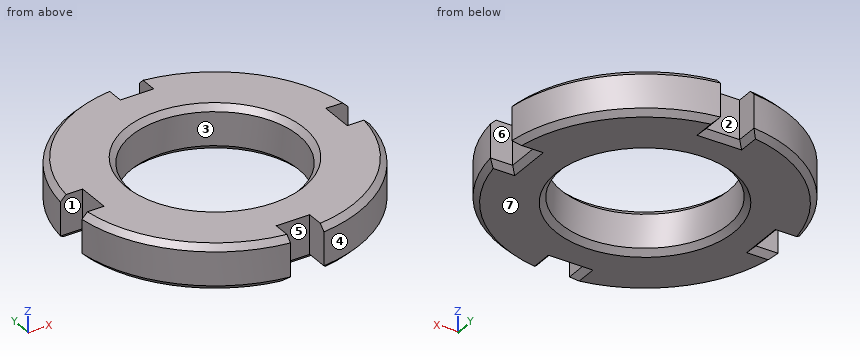
```python
from build123d import *

# Parameters (mm, degrees)
SKETCH_1_R      = 7.5
EXTRUDE_1_DEPTH = 4
CHAMFER_1_SIZE  = 0.5


with BuildPart() as part:
    # Эскиз1 → Бобышка-Вытянуть1 (new body)
    with BuildSketch(Plane.XY):
        with BuildLine():
            Line((1.5, 12.91317157), (1.5, 10.91317157))
            Line((1.5, 10.91317157), (-1.5, 10.91317157))
            Line((-1.5, 10.91317157), (-1.5, 12.91317157))
            ThreePointArc((-1.5, 12.91317157), (-9.192388155, 9.192388155), (-12.91317157, 1.5))
            Line((-12.91317157, 1.5), (-10.91317157, 1.5))
            Line((-10.91317157, 1.5), (-10.91317157, -1.5))
            Line((-10.91317157, -1.5), (-12.91317157, -1.5))
            ThreePointArc((-12.91317157, -1.5), (-9.192388155, -9.192388155), (-1.5, -12.91317157))
            Line((-1.5, -12.91317157), (-1.5, -10.91317157))
            Line((-1.5, -10.91317157), (1.5, -10.91317157))
            Line((1.5, -10.91317157), (1.5, -12.91317157))
            ThreePointArc((1.5, -12.91317157), (9.192388155, -9.192388155), (12.91317157, -1.5))
            Line((12.91317157, -1.5), (10.91317157, -1.5))
            Line((10.91317157, -1.5), (10.91317157, 1.5))
            Line((10.91317157, 1.5), (12.91317157, 1.5))
            ThreePointArc((12.91317157, 1.5), (9.192388155, 9.192388155), (1.5, 12.91317157))
        make_face()
        Circle(SKETCH_1_R, mode=Mode.SUBTRACT)
    extrude(amount=EXTRUDE_1_DEPTH)

    # Фаска1
    chamfer_1_edges = [part.edges().sort_by_distance(p)[0] for p in [
        (-1.5, 11.91317157, 0),
        (0, 10.91317157, 0),
        (1.5, 11.91317157, 0),
        (9.192388155, 9.192388155, 0),
        (11.91317157, 1.5, 0),
        (-9.192388155, -9.192388155, 4),
        (10.91317157, 0, 0),
        (11.91317157, -1.5, 0),
        (9.192388155, -9.192388155, 0),
        (1.5, -11.91317157, 0),
        (0, -10.91317157, 0),
        (-1.5, -11.91317157, 0),
        (-9.192388155, -9.192388155, 0),
        (-11.91317157, -1.5, 0),
        (-10.91317157, 0, 0),
        (-11.91317157, 1.5, 0),
        (-9.192388155, 9.192388155, 0),
        (9.192388155, -9.192388155, 4),
        (-7.5, 0, 0),
        (-7.5, 0, 4),
        (-9.192388155, 9.192388155, 4),
        (9.192388155, 9.192388155, 4),
    ]]
    chamfer(chamfer_1_edges, length=CHAMFER_1_SIZE)


solid = part.part
```
Can you work these out from the model? Positions are in its coordinate system, mm. Face numbers are marked on the shaded views. A direction names the side the tool comes from. Coordinates: 2 decimals unless noted, no trailing zeros. Loops run counter-clockwise (first coordinate to the right, second up) from the corner with the lowest first, then second, coordinate; pieces in that order, holes last. Notation, with made-up numbers: M 79.25,-31.75 L 121.25,-31.75 A26 cw 121.25,-13.75 Z; hole C -28,78 d4. An arc over 180 degrees is marked long. Put each result on its own line as item: value. Start each with the question number.
(1) Will these pins go through, and if not, where does the flat tip stop? pin 1 Ø1 at (x, z) = (11.5, 1.5) entering from -Y; pin 2 Ø1 at (x, z) = (-2.5, 3) entering from -Y; pin 3 Ø1.6 at (x, z) = (-12.5, 2) entering from -Y; pin 4 Ø12 at (x, y) = (-8.5, 4.5) entering from -Z.
(2) We'd pull the mould along X, two halves only. Please class the marked faces 1, 2, 3 and 4: +X half, -X half, draft (parallel to the pull), parting line (faces both ways), or undercut.
(3) Which directions (+Z, -Z, +X, -X, +Y, -Y) give clear straight access to the entire face, cutting with the end or side of a thin tool? Please do the marked faces 5, 6 and 7.
(4) Imagine slicing it at B-B on z = 2.6. List the corners of the cut face in (x, y) for me, and give its area (3 significant figures).
(5) Imagine slicing it at A-A on y = 0. List the corners of the cut face in (x, z) for me.
(6) I need wall thicknesses on probe 1 along Y at (x, z) = (0, 2.55); probe 2 along X at (y, z) = (0.75, 2.35); probe 3 along X at (y, z) = (-5, 1.3). Which ranges of each line are inside material? Lowest first, please.
Worked answers:
1. pin 1: stops at y = -6.93
1. pin 2: stops at y = -12.85
1. pin 3: stops at y = -5.67
1. pin 4: stops at z = 0
2. face 1: draft
2. face 2: undercut
2. face 3: undercut
2. face 4: +X half
3. face 5: +Z, -Z, -Y
3. face 6: +Z, -Z, +X
3. face 7: -Z, +X, -X, +Y, -Y
4. outline: M -12.91,-1.5 A13 ccw -1.5,-12.91 L -1.5,-10.91 L 1.5,-10.91 L 1.5,-12.91 A13 ccw 12.91,-1.5 L 10.91,-1.5 L 10.91,1.5 L 12.91,1.5 A13 ccw 1.5,12.91 L 1.5,10.91 L -1.5,10.91 L -1.5,12.91 A13 ccw -12.91,1.5 L -10.91,1.5 L -10.91,-1.5 Z; hole C 0,0 d15
4. area: 330 mm2
5. outline: M -10.91,0.5 L -10.41,0 L -8,0 L -7.5,0.5 L -7.5,3.5 L -8,4 L -10.91,4 Z; M 7.5,0.5 L 8,0 L 10.41,0 L 10.91,0.5 L 10.91,4 L 8,4 L 7.5,3.5 Z
6. probe 1: y = -10.91 to -7.5, 7.5 to 10.91
6. probe 2: x = -10.91 to -7.46, 7.46 to 10.91
6. probe 3: x = -12 to -5.59, 5.59 to 12
